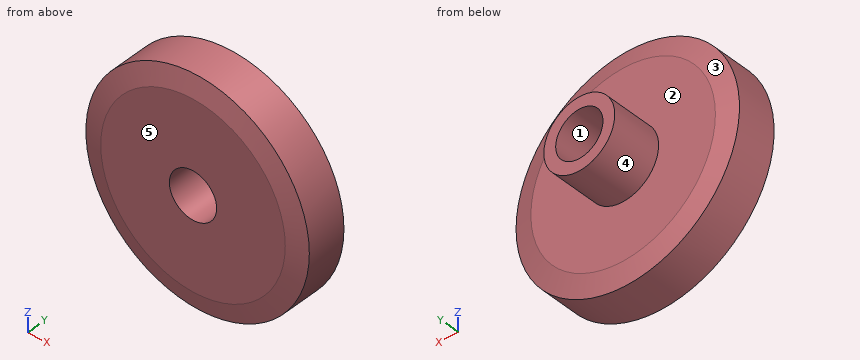
from build123d import *

# Parameters (mm, degrees)
CHAMFER_2_SIZE           = 1.645
CHAMFER_2_SIZE2          = 0.440776422
CHAMFER_3_SIZE           = 1.645
CHAMFER_3_SIZE2          = 0.440776422
SKETCH_4_R               = 2
CUT_EXTRUDE_2_DEPTH      = 1
CUT_EXTRUDE_2_DEPTH_BACK = 9.4


with BuildPart() as part:
    # Эскиз2 → Повернуть2 (revolve)
    with BuildSketch(Plane.XY):
        Polygon((0, 0), (9.45, 0), (9.45, 4.2), (3, 4.2), (3, 8.4), (0, 8.4), align=None)
    revolve(axis=Axis((0, 8.4, 0), (0, -1, 0)))

    # Фаска2
    chamfer_2_edges = [part.edges().sort_by_distance(p)[0] for p in [
        (-9.45, 4.2, 0),
    ]]
    chamfer_2_side = [part.faces().sort_by_distance(p)[0] for p in [
        (-9.182713637, 4.2, 0),
    ]]
    chamfer(chamfer_2_edges, length=CHAMFER_2_SIZE, length2=CHAMFER_2_SIZE2, reference=chamfer_2_side[0])

    # Фаска3
    chamfer_3_edges = [part.edges().sort_by_distance(p)[0] for p in [
        (-9.45, 0, 0),
    ]]
    chamfer_3_side = [part.faces().sort_by_distance(p)[0] for p in [
        (0, 0, 0),
    ]]
    chamfer(chamfer_3_edges, length=CHAMFER_3_SIZE, length2=CHAMFER_3_SIZE2, reference=chamfer_3_side[0])

    # Эскиз4 → Вырез-Вытянуть2 (cut, two sides)
    with BuildSketch(Plane(origin=(0, 8.4, 0), x_dir=(1, 0, 0), z_dir=(0, 1, 0))) as cut_extrude_2_sk:
        Circle(SKETCH_4_R)
    extrude(amount=CUT_EXTRUDE_2_DEPTH, mode=Mode.SUBTRACT)
    extrude(cut_extrude_2_sk.sketch, amount=-CUT_EXTRUDE_2_DEPTH_BACK, mode=Mode.SUBTRACT)


solid = part.part
Can you work these out from the model? Positions are in its coordinate system, mm. Face numbers are marked on the shaded views. A direction names the side the tool comes from. Coordinates: 2 decimals unless noted, no trailing zeros. Write each loop counter-clockwise with the first axis right and the second up, starting at its lowest first coordinate (ties: lowest second). Pieces come first, ordered by that corner, then holes. Notation, with made-up numbers: (-0.5, 53.25) -> (29.5, 53.25) arc R38 ccw to (29.5, 91.25) -> close; hole circle Ø10 at (42.25, 58.5). An arc over 180 degrees is marked (long way). Answer as CSV lines item,"result".
1) If we mould it in two halves opening along X, with no side actions, what happens to the marked faces 1, 2 and 3? For each: +X half, -X half, draft (parallel to the pull), parting line (faces both ways), or undercut.
Check result:
face 1,"undercut"
face 2,"draft"
face 3,"parting line"
2) On a 3-axis mill with a long thin cutter (end or side, diameter ignored), from which of +Z, -Z, +X, -X, +Y, -Y can I reach the whole of each face in a straight line? I mean the marked faces 4 and 5. Say none if no direction works.
Check result:
face 4,"+Y"
face 5,"+Z, -Z, +X, -X, -Y"
3) Will these pins go through, and if not, where does the flat tip stop? P1, Ø1, axis at y = 3, z = -6, coming from the -X side; P2, Ø2, axis at x = 5, y = 3.5, coming from the -Z side; P3, Ø2, axis at y = 3, z = -6, coming from the -X side.
Check result:
P1,"x = -7.68"
P2,"z = -8.56"
P3,"x = -8.02"
4) If we section it at A-A on z = 0: Please give me the cut outline in (x, y) (3 decimals), then the cut area to 3 significant figures.
Check result:
outline,"(-9.45, 0.441) -> (-7.805, 0) -> (-2, 0) -> (-2, 8.4) -> (-3, 8.4) -> (-3, 4.2) -> (-7.805, 4.2) -> (-9.45, 3.759) -> close; (2, 0) -> (7.805, 0) -> (9.45, 0.441) -> (9.45, 3.759) -> (7.805, 4.2) -> (3, 4.2) -> (3, 8.4) -> (2, 8.4) -> close"
area,"69.5 mm²"
5) If we section it at C-C on y = 1.25: Please give me the cut outline in (x, z), then the cut area to 3 significant figures.
Check result:
outline,"circle Ø18.9 at (0, 0); hole circle Ø4 at (0, 0)"
area,"268 mm²"
6) If we section it at D-D on y = 6.5: Please give me the cut outline in (x, z).
Check result:
outline,"circle Ø6 at (0, 0); hole circle Ø4 at (0, 0)"
7) If we section it at B-B on x = 0: Please give me the cut outline in (y, z) (3 decimals), then the cut area to 3 significant figures.
Check result:
outline,"(0, -7.805) -> (0.441, -9.45) -> (3.759, -9.45) -> (4.2, -7.805) -> (4.2, -3) -> (8.4, -3) -> (8.4, -2) -> (0, -2) -> close; (0, 2) -> (8.4, 2) -> (8.4, 3) -> (4.2, 3) -> (4.2, 7.805) -> (3.759, 9.45) -> (0.441, 9.45) -> (0, 7.805) -> close"
area,"69.5 mm²"
8) If I drill on line 1 (Z direction, x = 0, y = 5); line 2 (Y direction, x = -4.75, z = 1.75); line 3 (Z direction, x = 0, y = 3.5), over which ranges is the centre line in solid material (lowest first)? Write a range as from..to.
Check result:
line 1,"-3..-2, 2..3"
line 2,"0..4.2"
line 3,"-9.45..-2, 2..9.45"
